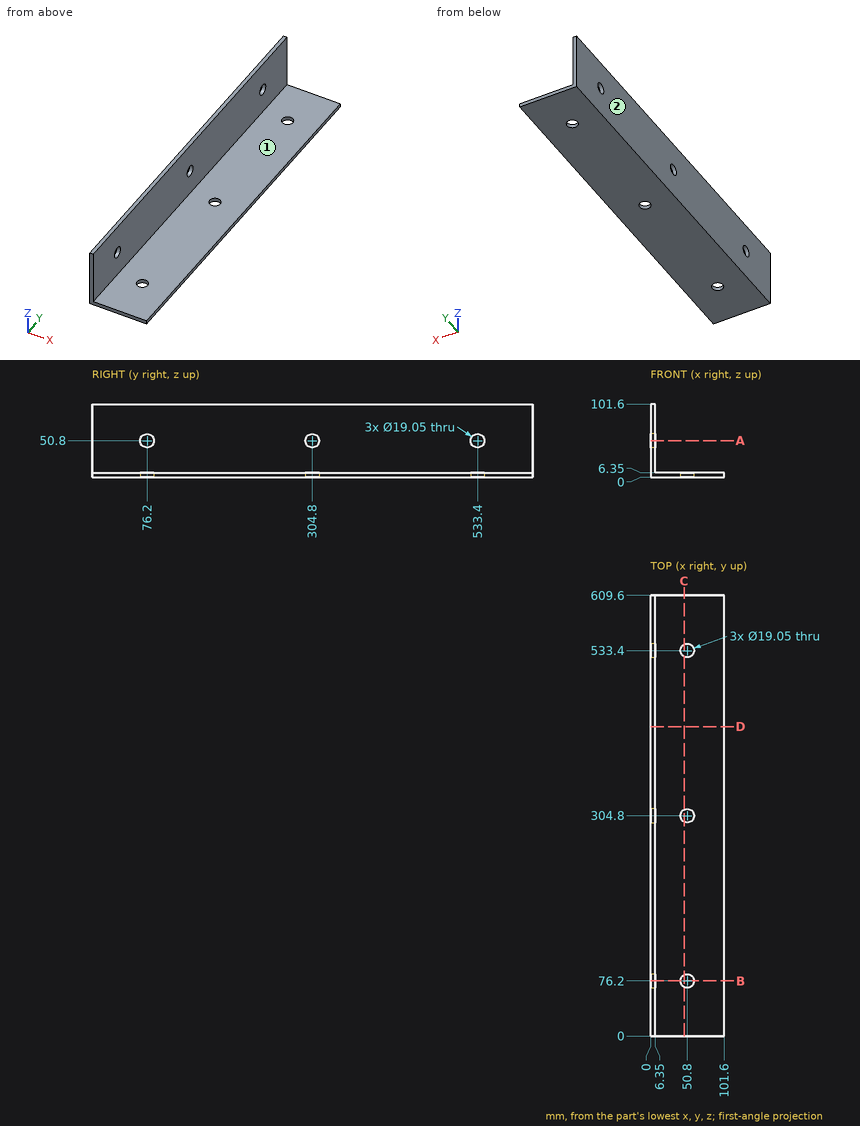
Print and shaded views of the part. All mm, measured from the part's lowest x, y and z. A direction names the side the tool comes from. Round coordinates to 2 decimals unless told otherwise and drop trailing zeros. Write each loop counter-clockwise with the first axis right and the second up, starting at its lowest first coordinate (ties: lowest second). Pieces come first, ordered by that corner, then holes. Notation, with made-up numbers: (-19.75, 19.5) -> (-6.75, 19.5) arc R25 cw to (-6.75, 39.5) -> close; hole circle Ø2 at (37, -33.5). An arc over 180 degrees is marked (long way). Answer in a Markdown table with one row per item. Add a question column.
Item 1: Saw through at B-B, the plane y = 76.2. Write the cut outline in (x, z) (3 decimals).
Item 2: Drill centre lines: line 1 (Y direction, x = 50.8, z = 4.5) (3 decimals); line 2 (X direction, y = 76, z = 3). Where is each one in solid material? Low to high. Write a range as from..to.
Item 3: Drop flat-ended pins along their axis: pin 1 Ø2 at (x, y) = (69, 63.5) entering from +Z; pin 2 Ø11.5 at (x, y) = (50.8, 76.2) entering from -Z; pin 3 Ø22 at (x, y) = (50.8, 533.4) entering from -Z. Give the stop position or say it passes through.
Item 4: Saw through at A-A, the plane z = 50.8. Write the cut outline in (x, y) (3 decimals), then the cut area to 3 significant figures.
Item 5: Saw through at D-D, the plane y = 428. Write the cut outline in (x, z), then the cut area to 3 significant figures.
Item 6: Which spindle directions (+Z, -Z, +X, -X, +Y, -Y) get a long thin tool onto all of the face, cutting with end or side? Do the marked faces 1 and 2. Say none if no direction does.
Item 7: Saw through at C-C, the plane x = 46.5. Write the cut outline in (y, z), then the cut area to 3 significant figures.
Findings below:
| question | item | result |
|---|---|---|
| 1 | outline | (0, 0) -> (41.275, 0) -> (41.275, 6.35) -> (6.35, 6.35) -> (6.35, 41.275) -> (0, 41.275) -> close; (0, 60.325) -> (6.35, 60.325) -> (6.35, 101.6) -> (0, 101.6) -> close; (60.325, 0) -> (101.6, 0) -> (101.6, 6.35) -> (60.325, 6.35) -> close |
| 2 | line 1 | y = 0..66.675, 85.725..295.275, 314.325..523.875, 542.925..609.6 |
| 2 | line 2 | x = 0..41.28, 60.32..101.6 |
| 3 | pin 1 | stops at z = 6.35 |
| 3 | pin 2 | passes through |
| 3 | pin 3 | stops at z = 0 |
| 4 | outline | (0, 0) -> (6.35, 0) -> (6.35, 66.675) -> (0, 66.675) -> close; (0, 85.725) -> (6.35, 85.725) -> (6.35, 295.275) -> (0, 295.275) -> close; (0, 314.325) -> (6.35, 314.325) -> (6.35, 523.875) -> (0, 523.875) -> close; (0, 542.925) -> (6.35, 542.925) -> (6.35, 609.6) -> (0, 609.6) -> close |
| 4 | area | 3,510 mm^2 |
| 5 | outline | (0, 0) -> (101.6, 0) -> (101.6, 6.35) -> (6.35, 6.35) -> (6.35, 101.6) -> (0, 101.6) -> close |
| 5 | area | 1,250 mm^2 |
| 6 | face 1 | +Z, +X, +Y, -Y |
| 6 | face 2 | +Z, -Z, -X, +Y, -Y |
| 7 | outline | (0, 0) -> (67.7, 0) -> (67.7, 6.35) -> (0, 6.35) -> close; (84.7, 0) -> (296.3, 0) -> (296.3, 6.35) -> (84.7, 6.35) -> close; (313.3, 0) -> (524.9, 0) -> (524.9, 6.35) -> (313.3, 6.35) -> close; (541.9, 0) -> (609.6, 0) -> (609.6, 6.35) -> (541.9, 6.35) -> close |
| 7 | area | 3,550 mm^2 |
